from build123d import *

# Parameters (mm, degrees)
SKETCH_1_W              = 94
SKETCH_1_H              = 72
EXTRUDE_1_DEPTH         = 2
SKETCH_2_W              = 8
SKETCH_2_H              = 10
EXTRUDE_2_DEPTH         = 2
FILLET_4_R              = 2
FILLET_5_R              = 2
SKETCH_3_R              = 1.5
CUT_EXTRUDE_1_DEPTH     = 90.716219269
SKETCH_4_W              = 64
SKETCH_4_H              = 2
EXTRUDE_3_DEPTH         = 45
FILLET_6_R              = 2
CONG_2_R                = 2
ENL_V_MAT_EXTRU_1_DEPTH = 66.833122363
CONG_3_R                = 3


with BuildPart() as part:
    # Эскиз1 → Бобышка-Вытянуть1 (new body)
    with BuildSketch(Plane(origin=(0, 0, 0), x_dir=(1, 0, 0), z_dir=(0, 1, 0))):
        Rectangle(SKETCH_1_W, SKETCH_1_H)
    extrude(amount=EXTRUDE_1_DEPTH)

    # Эскиз2 → Бобышка-Вытянуть2 (add)
    with BuildSketch(Plane.XY.offset(36)):
        with Locations((-28, -3)):
            Rectangle(SKETCH_2_W, SKETCH_2_H)
        with Locations((28, -3)):
            Rectangle(SKETCH_2_W, SKETCH_2_H)
        with Locations((0, -3)):
            Rectangle(SKETCH_2_W, SKETCH_2_H)
    extrude_2 = extrude(amount=EXTRUDE_2_DEPTH)

    # Скругление4
    fillet_4_edges = [part.edges().sort_by_distance(p)[0] for p in [
        (-24, 1, 36),
        (32, 1, 36),
        (4, 1, 36),
        (24, 1, 36),
        (-4, 1, 36),
        (-32, 1, 36),
    ]]
    fillet(fillet_4_edges, radius=FILLET_4_R - 0.0001)  # a hair under: the kernel refuses the full size

    # Зеркальное отражение1: Бобышка-Вытянуть2 across plane
    add(extrude_2.mirror(Plane.XY))

    # Скругление5
    fillet_5_edges = [part.edges().sort_by_distance(p)[0] for p in [
        (24, 1, -36),
        (-4, 1, -36),
        (-32, 1, -36),
        (-24, 1, -36),
        (4, 1, -36),
        (32, 1, -36),
    ]]
    fillet(fillet_5_edges, radius=FILLET_5_R - 0.0001)  # a hair under: the kernel refuses the full size

    # Эскиз3 → Вырез-Вытянуть1 (cut, through all)
    with BuildSketch(Plane(origin=(0, 0, -38), x_dir=(-1, 0, 0), z_dir=(0, 0, -1))):
        with Locations((-28, -4)):
            Circle(SKETCH_3_R)
        with Locations((0, -4)):
            Circle(SKETCH_3_R)
        with Locations((28, -4)):
            Circle(SKETCH_3_R)
    extrude(amount=-CUT_EXTRUDE_1_DEPTH, mode=Mode.SUBTRACT)

    # Эскиз4 → Бобышка-Вытянуть3 (add, symmetric)
    with BuildSketch(Plane(origin=(0, 0, 0), x_dir=(-1, 0, 0), z_dir=(0, 0, -1))):
        with Locations((0, 1)):
            Rectangle(SKETCH_4_W, SKETCH_4_H)
    extrude(amount=EXTRUDE_3_DEPTH, both=True)

    # Скругление6
    fillet_6_edges = [part.edges().sort_by_distance(p)[0] for p in [
        (-32, 1, 45),
        (32, 1, 45),
        (-32, 1, -45),
        (32, 1, -45),
    ]]
    fillet(fillet_6_edges, radius=FILLET_6_R)

    # Congé2
    cong_2_edges = [part.edges().sort_by_distance(p)[0] for p in [
        (47, 1, 36),
        (-47, 1, 36),
        (-47, 1, -36),
        (47, 1, -36),
    ]]
    fillet(cong_2_edges, radius=CONG_2_R)

    # Esquisse1 → Enlèv. mat.-Extru.1 (cut, through all)
    with BuildSketch(Plane(origin=(0, 2, 0), x_dir=(1, 0, 0), z_dir=(0, 1, 0))):
        Polygon((-47, -29), (-40, -36), (-47, -36), align=None)
        Polygon((-47, 36), (-40, 36), (-47, 29), align=None)
        Polygon((47, -29), (47, -36), (40, -36), align=None)
        Polygon((47, 29), (47, 36), (40, 36), align=None)
    extrude(amount=-ENL_V_MAT_EXTRU_1_DEPTH, mode=Mode.SUBTRACT)

    # Congé3
    cong_3_edges = [part.edges().sort_by_distance(p)[0] for p in [
        (-47, 1, -29),
        (-40, 1, -36),
        (40, 1, 36),
        (47, 1, 29),
        (47, 1, -29),
        (40, 1, -36),
        (-47, 1, 29),
        (-40, 1, 36),
    ]]
    fillet(cong_3_edges, radius=CONG_3_R)


solid = part.part
Work out the finished part from the listing and answer in its coordinate system (mm). A direction names the side the tool comes from. Round coordinates to 2 decimals unless told otherwise and drop trailing zeros. Order: outer loops, then holes, each group sorted by start corner. A loop starts at its lowest first (then second) coordinate and runs counter-clockwise, first axis right, second up. Notation, with made-up numbers: M 36,34.5 L 48,34.5 A13 ccw 48,42.5 Z; hole C 36.25,27.25 d2. An arc over 180 degrees is marked long. One line per item, written item: value.
Q1. Determine the mould class of faces 1 (the face through (29.5, -3.93, 36.99)), 2 (the face through (0, -8, -37)), 3 (the face through (32, 1, -41)) for opening direction Y: released by +Y, released by -Y, zero draft, split by the parting line, or undercut.
Derived:
face 1: undercut
face 2: released by -Y
face 3: zero draft
Q2. Flat-ended cylindrical pins translate along their axes: pin 1 (2.5 mm diameter, centred on x = -30, y = -3, fed in from -Z); pin 2 (10 mm diameter, centred on x = -30, z = -26, fed in from -Y); pin 3 (0.6 mm diameter, centred on y = -4.5, z = -37, fed in from +X). Find the tip coordinate at first contact, or state that the pin passes through.
Derived:
pin 1: z = -38
pin 2: y = 0
pin 3: x = 32
Q3. Find section C-C on x = -12. Write down the section's boundary in (y, z), then the cut area to 3 significant figures.
Derived:
outline: M 0,-45 L 2,-45 L 2,45 L 0,45 Z
area: 180 mm²
Q4. Find section B-B on y = -4. Give the number of separate pieces and of enclosed holes in the cut face, then the cut area to 3 significant figures.
Derived:
separate pieces: 12
enclosed holes: 0
area: 60.0 mm²
Q5. Straight lines are drawn through the part: line 1 (Z direction, x = -30.5, y = -4.5); line 2 (Y direction, x = -28, z = -36.85); line 3 (Y direction, x = 43.5, z = 22). For each, find the intervals that lie inside material, in ascending order.
Derived:
line 1: -38 to -36, 36 to 38
line 2: -8 to -5.5, -2.5 to 2
line 3: 0 to 2
Q6. Find section D-D on z = -2. Write down the section's boundary in (x, y).
Derived:
outline: M -47,0 L 47,0 L 47,2 L -47,2 Z
Q7. For faces 4 (the face through (-32, 1, 40)), 5 (the face through (-26, -4, 38)), 6 (the face through (0, -6, -38)), determine the directions among +Z, -Z, +X, -X, +Y, -Y from which every point of the face is accessible in a straight line to the end or side of a thin tool.
Derived:
face 4: +Z, -X, +Y, -Y
face 5: +Z, +X, -X, -Y
face 6: -Z, +X, -X, -Y
Q8. Find section A-A on x = 0. Write down the section's boundary in (y, z), then the cut area to 3 significant figures.
Derived:
outline: M -8,-38 L -5.5,-38 L -5.5,-36 L -8,-36 Z; M -8,36 L -5.5,36 L -5.5,38 L -8,38 Z; M -2.5,-38 L 0,-38 L 0,-45 L 2,-45 L 2,45 L 0,45 L 0,38 L -2.5,38 L -2.5,36 L 0,36 L 0,-36 L -2.5,-36 Z
area: 200 mm²
